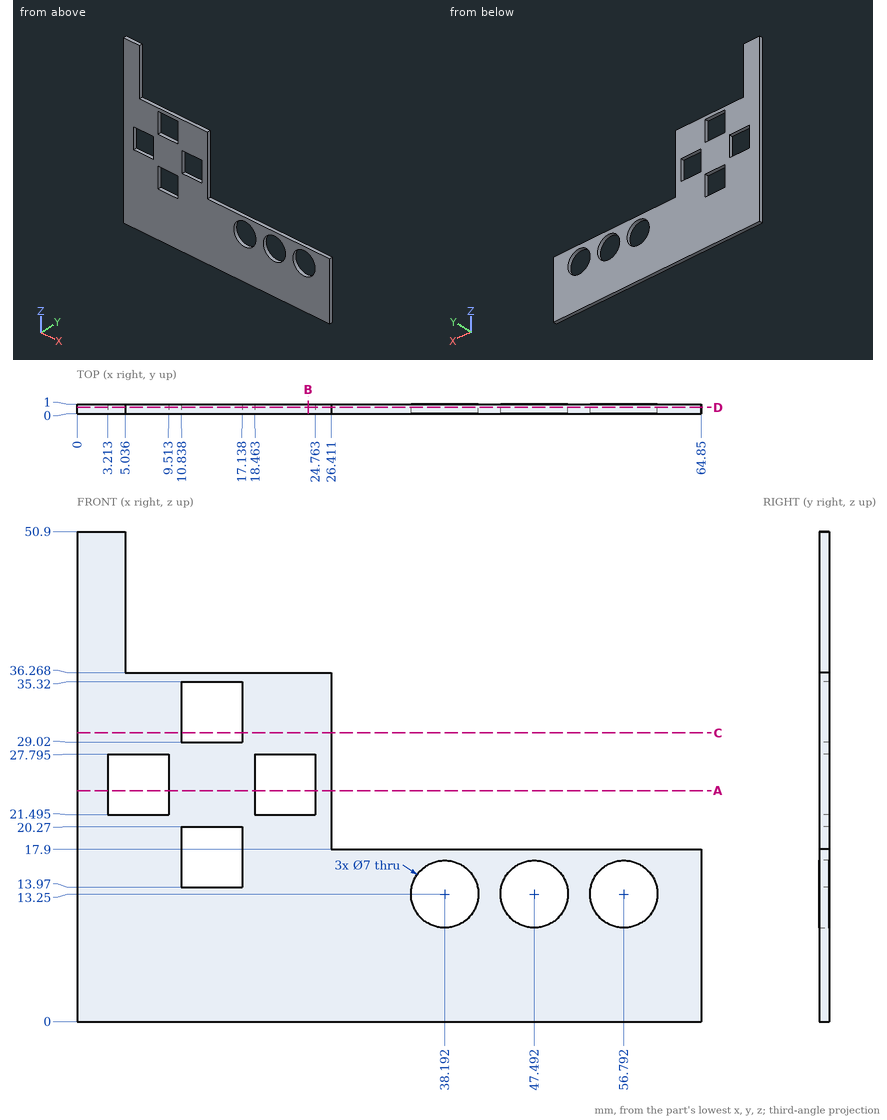
Answer from the drawing. Dimensions are ordinates in mm from the lowest x, y and z of the part. Coordinates: 2 decimals unless noted, no trailing zeros. Write each loop counter-clockwise with the first axis right and the second up, starting at its lowest first coordinate (ties: lowest second). Pieces come first, ordered by that corner, then holes. Notation, with made-up numbers: (-9, 79) - (36, 79) arc R21 cw to (36, 98) - close; hole circle Ø2 at (15, 75.25). An arc over 180 degrees is marked (long way). Return JSON: item names as keys, results as strings.
1. Each of these flat-tipped pins is pushed along its axis until it touches: pin 1 Ø0.5 at (y, z) = (0.5, 28) entering from +X; pin 2 Ø0.5 at (x, y) = (40.5, 0.5) entering from +Z. Where does it stop, or does it pass through?
Final values:
{"pin 1": "x = 26.41", "pin 2": "z = 17.9"}
2. The part is cut by section C-C on z = 30. Determine the outline of the cut face in (x, y), then the cut area to 3 significant figures.
Final values:
{"outline": "(0, 0) - (10.84, 0) - (10.84, 1) - (0, 1) - close; (17.14, 0) - (26.41, 0) - (26.41, 1) - (17.14, 1) - close", "area": "20.1 mm^2"}
3. The part is cut by section A-A on z = 24. Determine the outline of the cut face in (x, y).
Final values:
{"outline": "(0, 0) - (3.21, 0) - (3.21, 1) - (0, 1) - close; (9.51, 0) - (18.46, 0) - (18.46, 1) - (9.51, 1) - close; (24.76, 0) - (26.41, 0) - (26.41, 1) - (24.76, 1) - close"}
4. Consider line 1 along Z through (x, y) = (4, 0.6) (1 decimal); line 2 along X through (y, z) = (0.5, 26.5); line 3 along Z through (x, y) = (11.5, 0.75). Determine where each line is inside the solid, lowest interval first.
Final values:
{"line 1": "0 to 21.5, 27.8 to 50.9", "line 2": "0 to 3.21, 9.51 to 18.46, 24.76 to 26.41", "line 3": "0 to 13.97, 20.27 to 29.02, 35.32 to 36.27"}
5. The part is cut by section B-B on x = 24. Determine the outline of the cut face in (y, z) (1 decimal).
Final values:
{"outline": "(0, 0) - (1, 0) - (1, 21.5) - (0, 21.5) - close; (0, 27.8) - (1, 27.8) - (1, 36.3) - (0, 36.3) - close"}
6. The part is cut by section D-D on y = 0.65. Count the separate pieces of the cut face and the enclosed holes in it, then the cut area to 3 significant figures.
Final values:
{"separate pieces": "1", "enclosed holes": "7", "area": "1,450 mm^2"}
